```python
from build123d import *

# Parameters (mm, degrees)
BOSS_EXTRUDE1_DEPTH             = 5.6
BOSS_EXTRUDE2_DEPTH             = 2
BOSS_EXTRUDE2_DEPTH_BACK        = 2
SKETCH4_R                       = 0.95
CUT_EXTRUDE1_DEPTH              = 1.5
SKETCH4_4_R                     = 1
CUT_EXTRUDE2_DEPTH              = 0.5
SKETCH5_R                       = 0.95
CUT_EXTRUDE3_DEPTH              = 1.5
SKETCH5_3_R                     = 1
CUT_EXTRUDE4_DEPTH              = 0.5
BOSS_EXTRUDE3_REACH             = 22.624
SKETCH6_W                       = 0.966611368
SKETCH6_H                       = 1
BOSS_EXTRUDE4_START             = -1.2
SKETCH8_W                       = 0.7
SKETCH8_H                       = 4.583786921
BOSS_EXTRUDE4_DEPTH             = 2.4
BOSS_EXTRUDE5_REACH             = 22.624
SKETCH10_W                      = 0.7
SKETCH10_H                      = 14.923504875
BOSS_EXTRUDE5_DIRECTION_2_REACH = 22.624
SKETCH13_W                      = 7.333222736
SKETCH13_H                      = 6.9
CUT_EXTRUDE8_DEPTH              = 21.62373565
BOSS_EXTRUDE6_REACH             = 16.274
BOSS_EXTRUDE6_DIRECTION_2_REACH = 16.274
CUT_EXTRUDE9_START              = -4.626097
SKETCH14_W                      = 2.44
SKETCH14_H                      = 4.8
CUT_EXTRUDE9_DEPTH              = 4.626097
BOSS_EXTRUDE7_DEPTH             = 1.7
CUT_EXTRUDE10_DEPTH             = 16.595543228
SKETCH18_W                      = 2.44
SKETCH18_H                      = 0.1
CUT_EXTRUDE11_DEPTH             = 16.022577853
CUT_EXTRUDE12_DEPTH             = 16.022577853
CUT_EXTRUDE12_DEPTH_BACK        = 16.022577853
SKETCH20_W                      = 7.333222736
SKETCH20_H                      = 3.236091791
CUT_EXTRUDE13_DEPTH             = 2.5
SKETCH21_3_R                    = 0.95
CUT_EXTRUDE14_DEPTH             = 1.5
SKETCH21_4_R                    = 1.000336047
CUT_EXTRUDE15_DEPTH             = 0.5
SKETCH22_W                      = 2.65
SKETCH22_H                      = 1.15
CUT_EXTRUDE16_DEPTH             = 3.6
SKETCH28_W                      = 3.8
SKETCH28_H                      = 1.7
BOSS_EXTRUDE10_DEPTH            = 0.15


with BuildPart() as part:
    # Sketch1 → Boss-Extrude1 (new body)
    with BuildSketch(Plane.XY):
        Polygon((-1.2, 0), (-1.9, 0), (-1.9, 4.583786921), (-2.7, 6.276200005), (-2.7, 19.507291796), (-2, 19.507291796), (-2, 6.276200005), (-1.2, 4.583786921), align=None)
    extrude(amount=BOSS_EXTRUDE1_DEPTH)

    # Sketch3 → Boss-Extrude2 (add, two sides: drawn at the far end of the back side and taken through both)
    with BuildSketch(Plane.XY.offset(2.8).offset(-BOSS_EXTRUDE2_DEPTH_BACK)):
        with BuildLine():
            Line((-1.9, 0), (-3.666611368, 5.268840762))
            Line((-3.666611368, 5.268840762), (-3.666611368, 8.268840762))
            ThreePointArc((-3.666611368, 8.268840762), (-2.975877619, 8.638135643), (-2.7, 9.371200005))
            Line((-2.7, 9.371200005), (-2.7, 6.276200005))
            Line((-2.7, 6.276200005), (-1.9, 4.583786921))
            Line((-1.9, 4.583786921), (-1.9, 0))
        make_face()
    extrude(amount=BOSS_EXTRUDE2_DEPTH + BOSS_EXTRUDE2_DEPTH_BACK)

    # Sketch4 → Cut-Extrude1 (cut)
    with BuildSketch(Plane.ZY.offset(3.666611368)):
        with Locations(Location((3.3, 6.768840762, 0), (0, 0, 270))):
            Circle(SKETCH4_R)
    extrude(amount=-CUT_EXTRUDE1_DEPTH, mode=Mode.SUBTRACT)

    # Sketch4<4> → Cut-Extrude2 (cut)
    with BuildSketch(Plane.ZY.offset(3.666611368)):
        with Locations(Location((3.3, 6.768840762, 0), (0, 0, 270))):
            Circle(SKETCH4_4_R)
    extrude(amount=-CUT_EXTRUDE2_DEPTH, mode=Mode.SUBTRACT)

    # Sketch5 → Cut-Extrude3 (cut)
    with BuildSketch(Plane(origin=(-1.707984686, -0.572677236, 0), x_dir=(0, 0, 1), z_dir=(-0.9481240996322365, -0.3179004430581389, 0))):
        with Locations(Location((2.3, 4.661132282, 0), (0, 0, 270))):
            Circle(SKETCH5_R)
    extrude(amount=-CUT_EXTRUDE3_DEPTH, mode=Mode.SUBTRACT)

    # Sketch5<3> → Cut-Extrude4 (cut)
    with BuildSketch(Plane(origin=(-1.707984686, -0.572677236, 0), x_dir=(0, 0, 1), z_dir=(-0.9481240996322365, -0.3179004430581389, 0))):
        with Locations(Location((2.3, 4.661132282, 0), (0, 0, 270))):
            Circle(SKETCH5_3_R)
    extrude(amount=-CUT_EXTRUDE4_DEPTH, mode=Mode.SUBTRACT)

    # Sketch6 → Boss-Extrude3 (add, up to next)
    with BuildSketch(Plane(origin=(0, 19.507291796, 0), x_dir=(1, 0, 0), z_dir=(0, 1, 0)), mode=Mode.PRIVATE) as boss_extrude3_sk1:
        with Locations((-3.183305684, -2.8)):
            Rectangle(SKETCH6_W, SKETCH6_H)
    boss_extrude3_tool1 = extrude(boss_extrude3_sk1.sketch, amount=-BOSS_EXTRUDE3_REACH, mode=Mode.PRIVATE) - part.part
    add(boss_extrude3_tool1.solids().sort_by_distance((-3.183306, 19.507292, 2.8))[0])


with BuildPart() as body_2:
    # Mirror7: mirrored copy
    add(part.part.mirror(Plane(origin=(0, 0, 0), x_dir=(0, 0, 1), z_dir=(1, 0, 0))))


with BuildPart() as part_1:
    add(part.part)

    add(body_2.part)  # Boss-Extrude4 merges body 2
    # Sketch8 → Boss-Extrude4 (add)
    with BuildSketch(Plane(origin=(0, 0, 0), x_dir=(0, 0, -1), z_dir=(1, 0, 0)).offset(BOSS_EXTRUDE4_START)):
        with Locations((-5.25, 2.291893461)):
            Rectangle(SKETCH8_W, SKETCH8_H)
    extrude(amount=BOSS_EXTRUDE4_DEPTH)

    # Sketch10 → Boss-Extrude5 (add, up to next)
    with BuildSketch(Plane(origin=(0, 0, 0), x_dir=(0, 0, -1), z_dir=(1, 0, 0)), mode=Mode.PRIVATE) as boss_extrude5_sk1:
        with Locations((-5.25, 12.045539359)):
            Rectangle(SKETCH10_W, SKETCH10_H)
    boss_extrude5_tool1 = extrude(boss_extrude5_sk1.sketch, amount=BOSS_EXTRUDE5_REACH, mode=Mode.PRIVATE) - part_1.part
    add(boss_extrude5_tool1.solids().sort_by_distance((0, 12.045539, 5.25))[0])

    # Sketch10 → Boss-Extrude5 direction 2 (add, up to next)
    with BuildSketch(Plane(origin=(0, 0, 0), x_dir=(0, 0, -1), z_dir=(1, 0, 0)), mode=Mode.PRIVATE) as boss_extrude5_direction_2_sk1:
        with Locations((-5.25, 12.045539359)):
            Rectangle(SKETCH10_W, SKETCH10_H)
    boss_extrude5_direction_2_tool1 = extrude(boss_extrude5_direction_2_sk1.sketch, amount=-BOSS_EXTRUDE5_DIRECTION_2_REACH, mode=Mode.PRIVATE) - part_1.part
    add(boss_extrude5_direction_2_tool1.solids().sort_by_distance((0, 12.045539, 5.25))[0])

    # Sketch13 → Cut-Extrude8 (cut, through all)
    with BuildSketch(Plane.XY.offset(5.6)):
        with Locations((0, 16.057291796)):
            Rectangle(SKETCH13_W, SKETCH13_H)
    extrude(amount=-CUT_EXTRUDE8_DEPTH, mode=Mode.SUBTRACT)

    # Boss-Extrude6: up to this face of the body (flat: up to its plane)
    boss_extrude6_end = Plane(part_1.part.faces().sort_by_distance((1.9, 2.291893461, 5.2))[0])
    # Sketch9 → Boss-Extrude6 (add, up to the picked face)
    with BuildSketch(Plane(origin=(0, 0, 0), x_dir=(0, 0, -1), z_dir=(1, 0, 0)), mode=Mode.PRIVATE) as boss_extrude6_sk1:
        Polygon((-5.58241188, 1.018611498), (-4.8, 0.201293385), (-4.8, -0.528706615), (-5.58241188, 0.288611498), align=None)
    boss_extrude6_tool1 = split(extrude(boss_extrude6_sk1.sketch, amount=BOSS_EXTRUDE6_REACH, mode=Mode.PRIVATE), bisect_by=boss_extrude6_end, keep=Keep.BOTH, mode=Mode.PRIVATE)
    add(boss_extrude6_tool1.solids().sort_by(Axis((0, 0.244952, 5.191206), (1, 0, 0)))[0])

    # Boss-Extrude6 direction 2: up to this face of the body (flat: up to its plane)
    boss_extrude6_direction_2_end = Plane(part_1.part.faces().sort_by_distance((-1.9, 2.291893461, 5.2))[0])
    # Sketch9 → Boss-Extrude6 direction 2 (add, up to the picked face)
    with BuildSketch(Plane(origin=(0, 0, 0), x_dir=(0, 0, -1), z_dir=(1, 0, 0)), mode=Mode.PRIVATE) as boss_extrude6_direction_2_sk1:
        Polygon((-5.58241188, 1.018611498), (-4.8, 0.201293385), (-4.8, -0.528706615), (-5.58241188, 0.288611498), align=None)
    boss_extrude6_direction_2_tool1 = split(extrude(boss_extrude6_direction_2_sk1.sketch, amount=-BOSS_EXTRUDE6_DIRECTION_2_REACH, mode=Mode.PRIVATE), bisect_by=boss_extrude6_direction_2_end, keep=Keep.BOTH, mode=Mode.PRIVATE)
    add(boss_extrude6_direction_2_tool1.solids().sort_by(Axis((0, 0.244952, 5.191206), (-1, 0, 0)))[0])

    # Sketch14 → Cut-Extrude9 (cut)
    with BuildSketch(Plane.XZ.offset(CUT_EXTRUDE9_START)):
        with Locations((0, 2.4)):
            Rectangle(SKETCH14_W, SKETCH14_H)
    extrude(amount=CUT_EXTRUDE9_DEPTH, mode=Mode.SUBTRACT)

    # Sketch16 → Boss-Extrude7 (add)
    with BuildSketch(Plane.XY.offset(5.6)):
        Polygon((-2.7, 12.607291796), (2.7, 12.607291796), (2.7, 6.276200005), (1.9, 4.583786921), (1.9, 2.833786921), (-1.9, 2.833786921), (-1.9, 4.583786921), (-2.7, 6.276200005), align=None)
    extrude(amount=BOSS_EXTRUDE7_DEPTH)

    # Sketch17 → Cut-Extrude10 (cut, through all)
    with BuildSketch(Plane.ZY.offset(1.9)):
        Polygon((4.8, -0.528706615), (4.8, 0), (5.6, 0.835690902), (5.6, 0), (5.306126476, 0), align=None)
    extrude(amount=-CUT_EXTRUDE10_DEPTH, mode=Mode.SUBTRACT)

    # Sketch18 → Cut-Extrude11 (cut, through all)
    with BuildSketch(Plane(origin=(0, 12.607291796, 0), x_dir=(1, 0, 0), z_dir=(0, 1, 0))):
        with Locations((0, -4.85)):
            Rectangle(SKETCH18_W, SKETCH18_H)
    extrude(amount=-CUT_EXTRUDE11_DEPTH, mode=Mode.SUBTRACT)

    # Sketch20 → Cut-Extrude12 (cut, two sides: drawn at the far end of the back side and taken through both)
    with BuildSketch(Plane.XY.offset(7.3).offset(-CUT_EXTRUDE12_DEPTH_BACK)):
        with Locations((0, 10.989245901)):
            Rectangle(SKETCH20_W, SKETCH20_H)
    extrude(amount=CUT_EXTRUDE12_DEPTH + CUT_EXTRUDE12_DEPTH_BACK, mode=Mode.SUBTRACT)

    # Sketch21 → Cut-Extrude13 (cut)
    with BuildSketch(Plane.ZY.offset(2.7)):
        with BuildLine():
            ThreePointArc((6.395601498, 8.251554659), (5.622145346, 8.169301503), (5.704398502, 7.395845352))
            Line((5.704398502, 7.395845352), (6.395601498, 8.251554659))
        make_face()
        with BuildLine():
            Line((6.395601498, 8.251554659), (5.704398502, 7.395845352))
            ThreePointArc((5.704398502, 7.395845352), (6.287085614, 7.327423458), (6.6, 7.823700005))
            ThreePointArc((6.6, 7.823700005), (6.546276548, 8.060785619), (6.395601498, 8.251554659))
        make_face()
    extrude(amount=-CUT_EXTRUDE13_DEPTH, mode=Mode.SUBTRACT)

    # Sketch21<3> → Cut-Extrude14 (cut)
    with BuildSketch(Plane.ZY.offset(2.7)):
        with Locations(Location((6.05, 7.823700005, 0), (0, 0, 270))):
            Circle(SKETCH21_3_R)
    extrude(amount=-CUT_EXTRUDE14_DEPTH, mode=Mode.SUBTRACT)

    # Sketch21<4> → Cut-Extrude15 (cut)
    with BuildSketch(Plane.ZY.offset(2.7)):
        with Locations(Location((6.05, 7.823700005, 0), (0, 0, 270))):
            Circle(SKETCH21_4_R)
    extrude(amount=-CUT_EXTRUDE15_DEPTH, mode=Mode.SUBTRACT)

    # Sketch22 → Cut-Extrude16 (cut)
    with BuildSketch(Plane(origin=(0, 9.371200005, 0), x_dir=(1, 0, 0), z_dir=(0, 1, 0))):
        with Locations((0.575, -6.1)):
            Rectangle(SKETCH22_W, SKETCH22_H)
    extrude(amount=-CUT_EXTRUDE16_DEPTH, mode=Mode.SUBTRACT)

    # Sketch28 → Boss-Extrude10 (add)
    with BuildSketch(Plane.XZ.offset(-2.833786921)):
        with Locations((0, 6.45)):
            Rectangle(SKETCH28_W, SKETCH28_H)
    extrude(amount=BOSS_EXTRUDE10_DEPTH)


solid = part_1.part
```
Verification items for the finished model (mm, model axes). A direction names the side the tool comes from. Give positions to 0.01 mm unless a question says otherwise; leave off trailing zeros. Order: outer loops, then holes, each group sorted by start corner. A loop starts at its lowest first (then second) coordinate and runs counter-clockwise, first axis right, second up. Notation, with made-up numbers: (26, 47) -> (50, 47) arc R23 ccw to (50, 64) -> close; hole circle Ø11 at (-29.75, -29). An arc over 180 degrees is marked (long way). One line per item, written item: value.
(1) Sectioned sample at B-B on z = 6.05. Record the cut outline in (x, y), then the cut area to 3 significant figures.
Final values:
outline: (-2.7, 6.28) -> (-1.9, 4.58) -> (-1.9, 2.68) -> (1.9, 2.68) -> (1.9, 4.58) -> (2.7, 6.28) -> (2.7, 9.37) -> (1.9, 9.37) -> (1.9, 5.77) -> (-0.75, 5.77) -> (-0.75, 7.27) -> (-1.2, 7.27) -> (-1.2, 6.87) -> (-2.2, 6.87) -> (-2.2, 6.82) -> (-2.7, 6.82) -> close; (-2.7, 8.82) -> (-2.2, 8.82) -> (-2.2, 8.77) -> (-1.2, 8.77) -> (-1.2, 8.37) -> (-0.75, 8.37) -> (-0.75, 9.37) -> (-2.7, 9.37) -> close
area: 18.8 mm^2
(2) Gauge pin test, flat ends, axial feed: pin 1 (1 mm diameter, centred on y = 6, z = 6.5, fed in from +X); pin 2 (1.8 mm diameter, centred on y = 6.77, z = 3.3, fed in from +X); pin 3 (0.6 mm diameter, centred on y = 7.5, z = 6, fed in from -X). Record the tip position at first contact, or that the pin passes through.
Final values:
pin 1: x = 2.7
pin 2: x = 2.17
pin 3: x = -1.2
(3) Sectioned sample at C-C on x = 0.5. Record the cut outline in (y, z) (3 decimals), then the cut area to 3 significant figures.
Final values:
outline: (0.104, 4.9) -> (9.371, 4.9) -> (9.371, 5.525) -> (5.771, 5.525) -> (5.771, 6.675) -> (9.371, 6.675) -> (9.371, 7.3) -> (2.684, 7.3) -> (2.684, 5.6) -> (0.836, 5.6) -> close
area: 13.5 mm^2
(4) Tool access check on faces 4 (the face through (2.67, 5.89, 2.94)), 5 (the face through (-3, 5, 4.8)), 6 (the face through (2.983, 8.63, 4.04)), 7 (the face through (-2, 8, 2)), 8 (the face through (2.983, 8.63, 1.539)). Record the directions out of +Z, -Z, +X, -X, +Y, -Y that give a thin tool (end or side, any length) a straight path to the whole face; none if there is none.
Final values:
face 4: +X
face 5: +Z, -X, -Y
face 6: +Z, +X, +Y
face 7: -Z, +Y
face 8: -Z, +X, +Y
(5) Draft check along X on faces 1 (the face through (-0.75, 7, 6)), 2 (the face through (-2.7, 9, 6)), 3 (the face through (3.42, 5.845, 2.917)). Enter one of: pulls with the +X half, pulls with the -X half, needs draft (parallel to the pull), parting line crosses it, or undercut.
Final values:
face 1: undercut
face 2: pulls with the -X half
face 3: needs draft
(6) Sectioned sample at A-A on z = 4.5. Record the cut outline in (x, y).
Final values:
outline: (-3.67, 5.27) -> (-1.9, 0) -> (-1.22, 0) -> (-1.22, 4.63) -> (-2, 6.28) -> (-2, 9.37) -> (-2.7, 9.37) arc R1.11 cw to (-3.67, 8.27) -> close; (1.22, 0) -> (1.9, 0) -> (3.67, 5.27) -> (3.67, 8.27) arc R1.11 cw to (2.7, 9.37) -> (2, 9.37) -> (2, 6.28) -> (1.22, 4.63) -> close
(7) Scan lines: line 1 along Z through (x, y) = (-2.25, 7.25); line 2 along Z through (x, y) = (1.5, 6.5) (3 decimals); line 3 along X through (y, z) = (0.5, 2.75). Record each from-to range of solid material in increasing order. Write a range as [from, to].
Final values:
line 1: [0, 2.48], [4.12, 5.23], [6.87, 7.3]
line 2: [4.9, 5.525], [6.675, 7.3]
line 3: [-2.07, -1.22], [1.22, 2.07]
(8) Sectioned sample at D-D on y = 1. Record the cut outline in (x, z).
Final values:
outline: (-2.24, 0.8) -> (-1.9, 0.8) -> (-1.9, 0) -> (-1.22, 0) -> (-1.22, 4.9) -> (1.22, 4.9) -> (1.22, 0) -> (1.9, 0) -> (1.9, 0.8) -> (2.24, 0.8) -> (2.24, 4.8) -> (1.9, 4.8) -> (1.9, 5.6) -> (-1.9, 5.6) -> (-1.9, 4.8) -> (-2.24, 4.8) -> close
